Input: dimensioned drawing with shaded views. Units: mm. Origin: part minimum x, y, z. A direction names the side the tool comes from. Give positions to 0.01 mm unless a question says otherwise; leave off trailing zeros. Order: outer loops, then holes, each group sorted by start corner. A loop starts at its lowest first (then second) coordinate and runs counter-clockwise, first axis right, second up. Notation, with made-up numbers: (80, 75) -> (95, 75) arc R33 ccw to (95, 108) -> close; hole circle Ø2 at (49.5, 86). An arc over 180 degrees is marked (long way). Use CSV: the item, a comma, the result in double quotes.
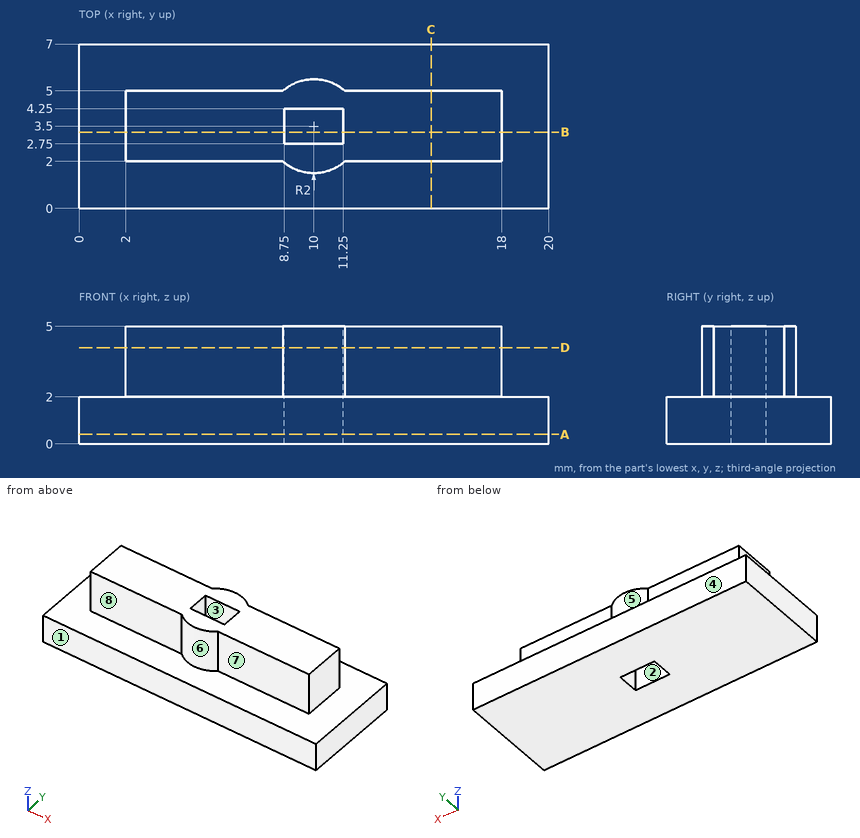
1. Mould query, pull axis Y, two halves, no side actions, for the marked faces 1, 2, 3 and 4. Classes: released by +Y, released by -Y, zero draft, split by the parting line, or undercut.
Answer below:
face 1,"released by -Y"
face 2,"undercut"
face 3,"undercut"
face 4,"released by +Y"
2. Ray query, line 1 along X through (y, z) = (3, 2.35); line 2 along Y through (x, z) = (10, 4.65); line 3 along Z through (x, y) = (4.25, 5.75). Return the intervals inside material, ascending.
Answer below:
line 1,"x = 2 to 8.75, 11.25 to 18"
line 2,"y = 1.5 to 2.75, 4.25 to 5.5"
line 3,"z = 0 to 2"
3. Section query B-B on y = 3.25. Return loops of the section in (x, z), plus the area to 3 significant figures.
Answer below:
outline,"(0, 0) -> (8.75, 0) -> (8.75, 5) -> (2, 5) -> (2, 2) -> (0, 2) -> close; (11.25, 0) -> (20, 0) -> (20, 2) -> (18, 2) -> (18, 5) -> (11.25, 5) -> close"
area,"75.5 mm²"
4. Section query A-A on z = 0.4. Return loops of the section in (x, y), plus the area to 3 significant figures.
Answer below:
outline,"(0, 0) -> (20, 0) -> (20, 7) -> (0, 7) -> close; hole (8.75, 2.75) -> (11.25, 2.75) -> (11.25, 4.25) -> (8.75, 4.25) -> close"
area,"136 mm²"
5. Section query C-C on x = 15. Return loops of the section in (y, z).
Answer below:
outline,"(0, 0) -> (7, 0) -> (7, 2) -> (5, 2) -> (5, 5) -> (2, 5) -> (2, 2) -> (0, 2) -> close"
6. Pin query (flat end, axial travel): P1, Ø0.9, axis at x = 6.5, z = 4, coming from the -Y side; P2, Ø1.5, axis at y = 3.5, z = 3.5, coming from the -X side; P3, Ø0.8, axis at x = 9.5, z = 2.5, coming from the -Y side. Return the tip coordinate at first contact, or that it passes through.
Answer below:
P1,"stops at y = 2"
P2,"stops at x = 2"
P3,"stops at y = 1.5"
7. Section query D-D on z = 4.1. Return loops of the section in (x, y).
Answer below:
outline,"(2, 2) -> (8.68, 2) arc R2 ccw to (11.32, 2) -> (18, 2) -> (18, 5) -> (11.32, 5) arc R2 ccw to (8.68, 5) -> (2, 5) -> close; hole (8.75, 2.75) -> (11.25, 2.75) -> (11.25, 4.25) -> (8.75, 4.25) -> close"
8. Access query for the marked faces 5, 6, 7 and 8. Directions: +Z, -Z, +X, -X, +Y, -Y. A direction counts if a zero-diameter tool reaches every point of the face in a straight line with its end or side. Return the directions, or none.
Answer below:
face 5,"+Z, +Y"
face 6,"+Z, -Y"
face 7,"+Z, +X, -Y"
face 8,"+Z, -X, -Y"
